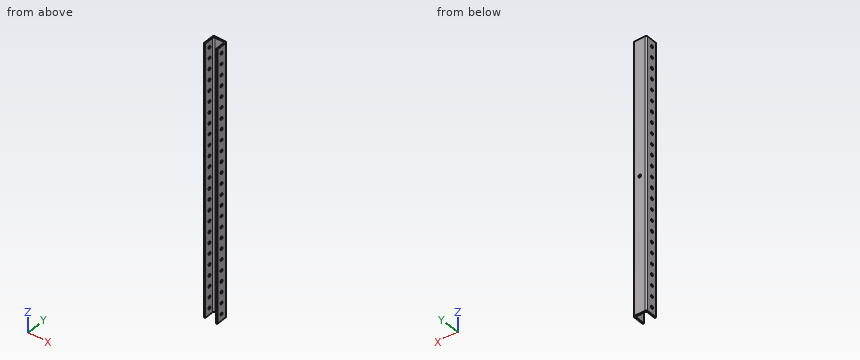
Autodesk Inventor part; units mm, degrees
ref_plane "YZ Plane" through (0, 0, 0) normal (1, 0, 0) x (0, 1, 0)
ref_plane "XZ Plane" through (0, 0, 0) normal (0, 1, 0) x (-1, 0, 0)
ref_plane "XY Plane" through (0, 0, 0) normal (0, 0, 1) x (1, 0, 0)
sketch "Sketch1" plane through (0, 0, 0) normal (0, 0, 1) x (1, 0, 0)
  line L0 (-15.875, 0) -> (-12.7, 0)
  line L1 (-12.7, 0) -> (-12.7, 22.352)
  line L2 (-9.525, 25.527) -> (9.525, 25.527)
  line L3 (12.7, 22.352) -> (12.7, 0)
  line L4 (12.7, 0) -> (15.875, 0)
  line L5 (15.875, 0) -> (15.875, 25.527)
  line L6 (12.7, 28.702) -> (-12.7, 28.702)
  line L7 (-15.875, 25.527) -> (-15.875, 0)
  arc A0 (-9.525, 25.527) -> (-12.7, 22.352) centre (-9.525, 22.352) ccw
  arc A1 (12.7, 22.352) -> (9.525, 25.527) centre (9.525, 22.352) ccw
  arc A2 (-12.7, 28.702) -> (-15.875, 25.527) centre (-12.7, 25.527) ccw
  arc A3 (15.875, 25.527) -> (12.7, 28.702) centre (12.7, 25.527) ccw
  line L8 (0, 35.2315) -> (0, -5.8719)
  point P0 (0, 0)
  dimension "d0" = 28.702
  dimension "d1" = 31.75
  dimension "d2" = 3.175
  dimension "d3" = 3.175
  dimension "d4" = 3.175
extrude "Extrusion1" add sketch "Sketch1" along normal mid plane 641.604
sketch "Sketch4" plane through (15.875, 0, 320.802) normal (1, 0, 0) x (0, 0, -1)
  line L0 (320.802, -5.7404) -> (320.802, 34.4424) construction
  line L1 (-128.3208, 0) -> (769.9248, 0) construction
  circle A0 centre (320.802, 12.7) radius 3.175
  point P0 (320.802, 0)
  dimension "d34" = 12.7
  dimension "d35" = 0
  dimension "d36" = 6.35
extrude "Extrusion4" cut sketch "Sketch4" against normal up to surface (31.75 mm away)
pattern_linear "Rectangular Pattern3" count 30 spacing 25.4 along (0, 0, 1) count 30 spacing 25.4 along (0, 0, -1) of "Extrusion4"
sketch "Sketch5" plane through (-12.7, 28.702, 320.802) normal (0, 1, 0) x (1, 0, 0)
  circle A0 centre (12.7, 320.802) radius 3.175
  dimension "d45" = 6.35
extrude "Extrusion5" cut sketch "Sketch5" against normal up to next
equation "\"d5\" = HingeLength"
equation "\"HingeLength\" = 641.604"
properties part number "NSupportChannel2"
Check sheet for the modelled part. Datum: model origin and axes. Units: mm. Give positions to 0.01 mm unless a question says otherwise; leave off trailing zeros. Order: outer loops, then holes, each group sorted by start corner. A loop starts at its lowest first (then second) coordinate and runs counter-clockwise, first axis right, second up. Notation, with made-up numbers: (-9.75, 41) -> (21.25, 41) arc R26 cw to (21.25, 66) -> close; hole circle Ø4 at (26, 30). An arc over 180 degrees is marked (long way). Return JSON: item names as keys, results as strings.
1. Go/stop test with flat-tipped pins: P1, Ø5, axis at y = 12.7, z = -101.6, coming from the +X side; P2, Ø1.5, axis at x = 1.5, z = 155, coming from the -Y side. Record where each tip stops, or that it passes through.
From the geometry:
{"P1": "through", "P2": "y = 25.53"}
2. Cross-section at A-A, the plane z = 168. Record the cut outline in (x, y) (3 decimals).
From the geometry:
{"outline": "(-15.875, 0) -> (-12.7, 0) -> (-12.7, 22.352) arc R3.175 cw to (-9.525, 25.527) -> (9.525, 25.527) arc R3.175 cw to (12.7, 22.352) -> (12.7, 0) -> (15.875, 0) -> (15.875, 25.527) arc R3.175 ccw to (12.7, 28.702) -> (-12.7, 28.702) arc R3.175 ccw to (-15.875, 25.527) -> close"}
3. Material ranges on probe 1 along X at (y, z) = (20.75, -58.5) (3 decimals); probe 2 along Y at (x, z) = (-13, 177); probe 3 along Y at (x, z) = (-13.6, 127) (3 decimals), recorded low to high. Write a range as [from, to].
From the geometry:
{"probe 1": "[-15.875, -12.7], [12.7, 15.875]", "probe 2": "[0, 9.63], [15.77, 28.69]", "probe 3": "[0, 9.525], [15.875, 28.572]"}
